For this review, take the finished solid that the model builds, in its own axes (mm). A direction names the side the tool comes from. Give positions to 0.01 mm unless a question says otherwise; leave off trailing zeros. Write each loop counter-clockwise with the first axis right and the second up, starting at its lowest first coordinate (ties: lowest second). Pieces come first, ordered by that corner, then holes. Notation, with made-up numbers: M 49,-25 L 104,-25 A25 cw 104,-11 Z; hole C 79.25,6.25 d1. An arc over 180 degrees is marked long. Write item = value, one per line.
```python
from build123d import *

# Parameters (mm, degrees)
F0_W      = 20.574
F0_H      = 20.574
F1_DEPTH  = 7.112
F2_W      = 17.018
F2_H      = 17.018
F3_DEPTH  = 5.334
F4_R      = 2.54
F5_W      = 5.588
F5_H      = 12.7
F6_DEPTH  = 3.048
F7_W      = 11.176
F7_H      = 12.7
F8_DEPTH  = 3.048
F9_R      = 0.3824187843
F9_R_2    = 0.3770429502
F10_DEPTH = 1.778
F11_R     = 1.27
F12_R     = 1.27


with BuildPart() as f1:
    # F0 (on Top) → F1 (new body)
    with BuildSketch(Plane.XY):
        Rectangle(F0_W, F0_H)
    extrude(amount=F1_DEPTH)

    # F2 (on face) → F3 (cut)
    with BuildSketch(Plane(origin=(0, 0, 0), x_dir=(1, 0, 0), z_dir=(0, 0, -1))):
        Rectangle(F2_W, F2_H)
    extrude(amount=-F3_DEPTH, mode=Mode.SUBTRACT)

    # F4
    f4_edges = [f1.edges().sort_by_distance(p)[0] for p in [
        (-10.287, -10.287, 3.556),
        (10.287, 10.287, 3.556),
        (10.287, -10.287, 3.556),
        (-10.287, 10.287, 3.556),
    ]]
    fillet(f4_edges, radius=F4_R)

    # F5 (on face) → F6 (cut)
    with BuildSketch(Plane.XY.offset(7.112)):
        with Locations((-7.493, 0)):
            Rectangle(F5_W, F5_H)
    extrude(amount=-F6_DEPTH, mode=Mode.SUBTRACT)

    # F7 (on face) → F8 (cut)
    with BuildSketch(Plane.XY.offset(7.112)):
        with Locations((10.287, 0)):
            Rectangle(F7_W, F7_H)
    extrude(amount=-F8_DEPTH, mode=Mode.SUBTRACT)

    # F9 (on face) → F10 (cut)
    with BuildSketch(Plane.XY.offset(7.112)):
        with Locations((-3.8157331292, 0)):
            Circle(F9_R)
        with Locations((3.8035737816, 0)):
            Circle(F9_R_2)
    extrude(amount=-F10_DEPTH, mode=Mode.SUBTRACT)

    # F11
    f11_edges = [f1.edges().sort_by_distance(p)[0] for p in [
        (0, 10.287, 7.112),
        (0, -10.287, 7.112),
    ]]
    fillet(f11_edges, radius=F11_R)

    # F12
    f12_edges = [f1.edges().sort_by_distance(p)[0] for p in [
        (-10.287, 0, 0),
        (0, 10.287, 0),
        (-9.543051, 9.543051, 0),
    ]]
    fillet(f12_edges, radius=F12_R)


solid = f1.part
```
1. Insertion check: P1, Ø2, axis at y = 2.5, z = 6, coming from the +X side; P2, Ø0.5, axis at x = -9.5, y = -2.5, coming from the +Z side; P3, Ø1, axis at x = 5.5, y = 6.5, coming from the -Z side. Each pin has a flat end and moves straight along its axis. Give the tip position at first contact, or say it passes through.
Responses:
P1 = 4.7
P2 = 4.06
P3 = 5.33
2. We need section C-C, the plane x = -0.75. Write out the cut boundary in (y, z).
Responses:
outline = M -10.29,1.27 A1.27 ccw -9.02,0 L -8.51,0 L -8.51,5.33 L 8.51,5.33 L 8.51,0 L 9.02,0 A1.27 ccw 10.29,1.27 L 10.29,5.84 A1.27 ccw 9.02,7.11 L -9.02,7.11 A1.27 ccw -10.29,5.84 Z
3. For line 1 along Y through (x, z) = (-2, 2.5); line 2 along Z through (x, y) = (-2.75, 1), list the stretches that pass through material, from the lowest coordinate up. Write a range as from..to.
Responses:
line_1 = -10.29..-8.51, 8.51..10.29
line_2 = 5.33..7.11
4. We need section B-B, the plane z = 3. Write out the cut boundary in (x, y), then the cut area to 3 significant figures.
Responses:
outline = M -10.29,-7.75 A2.54 ccw -7.75,-10.29 L 7.75,-10.29 A2.54 ccw 10.29,-7.75 L 10.29,7.75 A2.54 ccw 7.75,10.29 L -7.75,10.29 A2.54 ccw -10.29,7.75 Z; hole M -8.51,-8.51 L 8.51,-8.51 L 8.51,8.51 L -8.51,8.51 Z
area = 128 mm2
5. The part is to be moulded in two halves that separate along X. For faces 1 (the face through (0, 8.509, 3)), 2 (the face through (8, -6.35, 6)), 3 (the face through (9.523, 9.563, 3.588)), 4 (the face through (-9.925, 0.108, 0.382)), say which applies: +X half, -X half, draft (parallel to the pull), parting line (faces both ways), or undercut.
Responses:
face_1 = undercut
face_2 = draft
face_3 = +X half
face_4 = -X half
6. We need section A-A, the plane y = -1.25. Write out the cut boundary in (x, z).
Responses:
outline = M -10.29,1.27 A1.27 ccw -9.02,0 L -8.51,0 L -8.51,4.06 L -10.29,4.06 Z; M -4.7,5.33 L 4.7,5.33 L 4.7,7.11 L -4.7,7.11 Z; M 8.51,0 L 9.02,0 A1.27 ccw 10.29,1.27 L 10.29,4.06 L 8.51,4.06 Z
7. Machinability: for faces 5 (the face through (0, 0, 7.112)), 6 (the face through (-4.699, 0, 6)), 7 (the face through (-8, 6.35, 6)), which of the approach directions +Z, -Z, +X, -X, +Y, -Y give a long, thin tool a straight path to every point of the face, cutting with its end or side? Answer none if there is none.
Responses:
face_5 = +Z, +X, -X, +Y, -Y
face_6 = +Z, -Z, -X
face_7 = +Z, -X
